Input: part model. Units: mm. Frame: model coordinates. A direction names the side the tool comes from. Coordinates: 2 decimals unless noted, no trailing zeros. Write each loop counter-clockwise with the first axis right and the second up, starting at its lowest first coordinate (ties: lowest second). Pieces come first, ordered by that corner, then holes. Notation, with made-up numbers: M -8.5,-27.75 L 32.5,-27.75 A6 ccw 32.5,-20.75 Z; hole C 74.5,-39 d10. An arc over 180 degrees is marked long. Use one line per item in the form item = value.
from build123d import *

# Parameters (mm, degrees)
F1_DEPTH = 5


with BuildPart() as f1:
    # F0 (on Top) → F1 (new body)
    with BuildSketch(Plane.XY):
        with BuildLine():
            ThreePointArc((-0.5828427764, 0.3365044338), (-0.28, 0.4849742261), (0, 0.6730088677))
            ThreePointArc((0, 0.6730088677), (-0.7642906068, 1.6619651488), (-0.9517724896, 2.8976937602))
            ThreePointArc((-0.9517724896, 2.8976937602), (-1.525, 2.6413774815), (-2.0335901639, 2.2731060347))
            ThreePointArc((-2.0335901639, 2.2731060347), (-1.0571587356, 1.4928776558), (-0.5828427764, 0.3365044338))
        make_face()
        with BuildLine():
            ThreePointArc((-0.56, 0), (-0.5657172578, 0.1686394278), (-0.5828427764, 0.3365044338))
            ThreePointArc((-0.5828427764, 0.3365044338), (-1.8214493424, 0.169087493), (-2.9853626535, 0.6245877255))
            ThreePointArc((-2.9853626535, 0.6245877255), (-3.05, 0), (-2.9853626535, -0.6245877255))
            ThreePointArc((-2.9853626535, -0.6245877255), (-1.8214493424, -0.169087493), (-0.5828427764, -0.3365044338))
            ThreePointArc((-0.5828427764, -0.3365044338), (-0.5657172578, -0.1686394278), (-0.56, 0))
        make_face()
        with BuildLine():
            ThreePointArc((0.5828427764, -0.3365044338), (0.56, 0), (0.5828427764, 0.3365044338))
            ThreePointArc((0.5828427764, 0.3365044338), (0.28, 0.4849742261), (0, 0.6730088677))
            ThreePointArc((0, 0.6730088677), (-0.28, 0.4849742261), (-0.5828427764, 0.3365044338))
            ThreePointArc((-0.5828427764, 0.3365044338), (-0.5657172578, 0.1686394278), (-0.56, 0))
            ThreePointArc((-0.56, 0), (-0.5657172578, -0.1686394278), (-0.5828427764, -0.3365044338))
            ThreePointArc((-0.5828427764, -0.3365044338), (-0.28, -0.4849742261), (0, -0.6730088677))
            ThreePointArc((0, -0.6730088677), (0.28, -0.4849742261), (0.5828427764, -0.3365044338))
        make_face()
        with BuildLine():
            ThreePointArc((0.5828427764, 0.3365044338), (1.0571587356, 1.4928776558), (2.0335901639, 2.2731060347))
            ThreePointArc((2.0335901639, 2.2731060347), (1.525, 2.6413774815), (0.9517724896, 2.8976937602))
            ThreePointArc((0.9517724896, 2.8976937602), (0.9616909236, 2.7697061628), (0.965, 2.6413774815))
            ThreePointArc((0.965, 2.6413774815), (0.7107716789, 1.545282139), (0, 0.6730088677))
            ThreePointArc((0, 0.6730088677), (0.28, 0.4849742261), (0.5828427764, 0.3365044338))
        make_face()
        with BuildLine():
            ThreePointArc((2.9853626535, -0.6245877255), (3.0337976278, -0.3139617068), (3.05, 0))
            ThreePointArc((3.05, 0), (3.0337976278, 0.3139617068), (2.9853626535, 0.6245877255))
            ThreePointArc((2.9853626535, 0.6245877255), (1.8214493424, 0.169087493), (0.5828427764, 0.3365044338))
            ThreePointArc((0.5828427764, 0.3365044338), (0.56, 0), (0.5828427764, -0.3365044338))
            ThreePointArc((0.5828427764, -0.3365044338), (1.8214493424, -0.169087493), (2.9853626535, -0.6245877255))
        make_face()
        with BuildLine():
            ThreePointArc((0.9517724896, -2.8976937602), (1.525, -2.6413774815), (2.0335901639, -2.2731060347))
            ThreePointArc((2.0335901639, -2.2731060347), (1.0571587356, -1.4928776558), (0.5828427764, -0.3365044338))
            ThreePointArc((0.5828427764, -0.3365044338), (0.28, -0.4849742261), (0, -0.6730088677))
            ThreePointArc((0, -0.6730088677), (0.7107716789, -1.545282139), (0.965, -2.6413774815))
            ThreePointArc((0.965, -2.6413774815), (0.9616909236, -2.7697061628), (0.9517724896, -2.8976937602))
        make_face()
        with BuildLine():
            ThreePointArc((-0.9517724896, -2.8976937602), (-0.7642906068, -1.6619651488), (0, -0.6730088677))
            ThreePointArc((0, -0.6730088677), (-0.28, -0.4849742261), (-0.5828427764, -0.3365044338))
            ThreePointArc((-0.5828427764, -0.3365044338), (-1.0571587356, -1.4928776558), (-2.0335901639, -2.2731060347))
            ThreePointArc((-2.0335901639, -2.2731060347), (-1.525, -2.6413774815), (-0.9517724896, -2.8976937602))
        make_face()
    extrude(amount=F1_DEPTH)


solid = f1.part
(1) Section query C-C on x = 0.75. Return the cut outline in (y, z).
Computed:
outline = M -1.63,0 L -0.95,0 L -0.95,5 L -1.63,5 Z; M -0.28,0 L 0.28,0 L 0.28,5 L -0.28,5 Z; M 0.95,0 L 1.63,0 L 1.63,5 L 0.95,5 Z
(2) Line query: probe 1 along Y at (x, z) = (1.25, 2.8); probe 2 along X at (y, z) = (1.4, 3); probe 3 along X at (y, z) = (-2.55, 1.75). Output: solid intervals per line, ascending.
Computed:
probe_1 = -2.78 to -1.72, -0.17 to 0.17, 1.72 to 2.78
probe_2 = -0.99 to -0.63, 0.63 to 0.99
probe_3 = -1.67 to -0.96, 0.96 to 1.67
(3) First-contact query: pin 1 Ø1 at (x, z) = (1, 2.5) entering from -Y. Flat tip, straight axial feed; report the tip coordinate or a pass-through.
Computed:
pin_1 = -2.9
(4) Section query B-B on y = -0.85. Return the cut outline in (x, z), plus the area to 3 significant figures.
Computed:
outline = M -0.71,0 L -0.2,0 L -0.2,5 L -0.71,5 Z; M 0.2,0 L 0.71,0 L 0.71,5 L 0.2,5 Z
area = 5.05 mm^2
(5) Pull-direction query (Y, two-part tool) for faces 3 (the flat face through (0, 0, 5)), 4 (the cylindrical face through (-3.05, 0.01, 2.46)), 5 (the cylindrical face through (-1.05, -1.48, 2.46)), 6 (the cylindrical face through (1.517, -2.646, 2.465)); classes: pulls with the +Y half, pulls with the -Y half, needs draft (parallel to the pull), parting line crosses it, or undercut.
Computed:
face_3 = needs draft
face_4 = parting line crosses it
face_5 = undercut
face_6 = pulls with the -Y half
(6) Section query D-D on y = 2.05. Return the cut outline in (x, z).
Computed:
outline = M -1.64,0 L -0.89,0 L -0.89,5 L -1.64,5 Z; M 0.89,0 L 1.64,0 L 1.64,5 L 0.89,5 Z
(7) Set-up query: faces 1 (the cylindrical face through (-1.53, -2.64, 2.46)), 2 (the cylindrical face through (-1.804, 0.167, 2.465)). Return all of +Z, -Z, +X, -X, +Y, -Y with unobstructed straight access to the full face (end or side cutting, diameter ignored); none if empty.
Computed:
face_1 = +Z, -Z, -X, -Y
face_2 = +Z, -Z
